Build history of the part. All positions in model axes, mm. Round coordinates to 2 decimals unless told otherwise and drop trailing zeros. Order: outer loops, then holes, each group sorted by start corner. A loop starts at its lowest first (then second) coordinate and runs counter-clockwise, first axis right, second up. Notation, with made-up numbers: M -1.75,-20.5 L 12.25,-20.5 A29 ccw 12.25,10.5 Z; hole C -31.5,4 d3. An arc over 180 degrees is marked long. One line per item, written item: value. Start each with the question number.
Item 1: Band-saw the part on B-B, the plane x = -73.5. Write the cut outline in (y, z).
Item 2: Band-saw the part on D-D, the plane x = 74.5. Write the cut outline in (y, z).
Item 3: Band-saw the part on A-A, the plane y = 117.61. Write the cut outline in (x, z), then the cut area to 3 significant figures.
Item 4: Pin check, flat tips, straight feed: pin 1 (3.5 mm diameter, centred on x = 43.36, y = -61.74, fed in from -Z); pin 2 (5.5 mm diameter, centred on x = -92.5, y = 129.72, fed in from -Z). Stop position of each tip, or through.
Item 5: Probe L1, parallel to Y at x = 86, z = 0.1; L2, parallel to Y at x = 61, z = 0.1; L3, parallel to Y at x = 23, z = 0.05. List the from-to ranges inside material, lowest first.
Item 6: Band-saw the part on C-C, the plane z = 0.1. Give the number of separate pieces and of enclosed holes in the cut face, then the cut area to 3 significant figures.
```python
from build123d import *

# Parameters (mm, degrees)
F0_R     = 2.25
F0_R_2   = 1.75
F0_R_3   = 10.5
F0_R_4   = 4.25
F0_R_5   = 2.75
F0_R_6   = 15
F1_DEPTH = 0.254


with BuildPart() as f1:
    # F0 (on Top) → F1 (new body)
    with BuildSketch(Plane.XY):
        Polygon((-17.5, -150), (92.5, -150), (102.5, -140), (102.5, -8.17), (92.5, 1.83), (58.4225, 1.83), (-7.088235, 108.588235), (-48.5, 150), (-86.5, 150), (-102.5, 134), (-102.5, -60), (-92.5, -70), (-37.5, -70), (-27.5, -80), (-27.5, -140), align=None)
        with Locations((-10.96, -138.5)):
            Circle(F0_R, mode=Mode.SUBTRACT)
        with BuildLine():
            Line((-13.21, -87.3), (-13.21, -83.3))
            ThreePointArc((-13.21, -83.3), (-10.96, -81.05), (-8.71, -83.3))
            Line((-8.71, -83.3), (-8.71, -87.3))
            ThreePointArc((-8.71, -87.3), (-10.96, -89.55), (-13.21, -87.3))
        make_face(mode=Mode.SUBTRACT)
        with Locations((-92.5, -50.28)):
            Circle(F0_R_2, mode=Mode.SUBTRACT)
        with Locations((-67.5, -38.17)):
            Circle(F0_R_3, mode=Mode.SUBTRACT)
        with Locations((-92.5, -22.78)):
            Circle(F0_R_2, mode=Mode.SUBTRACT)
        with Locations((-42.5, -50.28)):
            Circle(F0_R_2, mode=Mode.SUBTRACT)
        with Locations((-13.07, -60.17)):
            Circle(F0_R_4, mode=Mode.SUBTRACT)
        with Locations((-42.5, -22.78)):
            Circle(F0_R_2, mode=Mode.SUBTRACT)
        with Locations((21.36, -138.5)):
            Circle(F0_R, mode=Mode.SUBTRACT)
        with BuildLine():
            Line((19.11, -87.3), (19.11, -83.3))
            ThreePointArc((19.11, -83.3), (21.36, -81.05), (23.61, -83.3))
            Line((23.61, -83.3), (23.61, -87.3))
            ThreePointArc((23.61, -87.3), (21.36, -89.55), (19.11, -87.3))
        make_face(mode=Mode.SUBTRACT)
        with Locations((53.68, -138.5)):
            Circle(F0_R, mode=Mode.SUBTRACT)
        with Locations((86, -138.5)):
            Circle(F0_R, mode=Mode.SUBTRACT)
        with BuildLine():
            Line((51.43, -87.3), (51.43, -83.3))
            ThreePointArc((51.43, -83.3), (53.68, -81.05), (55.93, -83.3))
            Line((55.93, -83.3), (55.93, -87.3))
            ThreePointArc((55.93, -87.3), (53.68, -89.55), (51.43, -87.3))
        make_face(mode=Mode.SUBTRACT)
        with BuildLine():
            Line((83.75, -87.3), (83.75, -83.3))
            ThreePointArc((83.75, -83.3), (86, -81.05), (88.25, -83.3))
            Line((88.25, -83.3), (88.25, -87.3))
            ThreePointArc((88.25, -87.3), (86, -89.55), (83.75, -87.3))
        make_face(mode=Mode.SUBTRACT)
        with Locations((21.93, -60.17)):
            Circle(F0_R_4, mode=Mode.SUBTRACT)
        with Locations((43.36, -61.74)):
            Circle(F0_R_5, mode=Mode.SUBTRACT)
        with Locations((43.36, -14.6)):
            Circle(F0_R_5, mode=Mode.SUBTRACT)
        with Locations((51.43, -53.67)):
            Circle(F0_R_2, mode=Mode.SUBTRACT)
        with Locations((66.93, -38.17)):
            Circle(F0_R_6, mode=Mode.SUBTRACT)
        with Locations((90.5, -61.74)):
            Circle(F0_R_5, mode=Mode.SUBTRACT)
        with Locations((82.43, -53.67)):
            Circle(F0_R_2, mode=Mode.SUBTRACT)
        with Locations((51.43, -22.67)):
            Circle(F0_R_2, mode=Mode.SUBTRACT)
        with Locations((82.43, -22.67)):
            Circle(F0_R_2, mode=Mode.SUBTRACT)
        with Locations((90.5, -14.6)):
            Circle(F0_R_5, mode=Mode.SUBTRACT)
        with Locations((-92.5, 4.72)):
            Circle(F0_R_2, mode=Mode.SUBTRACT)
        with Locations((-91.07, 16.15)):
            Circle(F0_R_5, mode=Mode.SUBTRACT)
        with Locations((-83, 24.22)):
            Circle(F0_R_2, mode=Mode.SUBTRACT)
        with Locations((-67.5, 4.72)):
            Circle(F0_R_2, mode=Mode.SUBTRACT)
        with Locations((-52, 24.22)):
            Circle(F0_R_2, mode=Mode.SUBTRACT)
        with Locations((-92.5, 39.72)):
            Circle(F0_R_2, mode=Mode.SUBTRACT)
        with Locations((-83, 55.22)):
            Circle(F0_R_2, mode=Mode.SUBTRACT)
        with Locations((-91.07, 63.29)):
            Circle(F0_R_5, mode=Mode.SUBTRACT)
        with Locations((-92.5, 74.72)):
            Circle(F0_R_2, mode=Mode.SUBTRACT)
        with Locations((-67.5, 39.72)):
            Circle(F0_R_6, mode=Mode.SUBTRACT)
        with Locations((-52, 55.22)):
            Circle(F0_R_2, mode=Mode.SUBTRACT)
        with Locations((-67.5, 74.72)):
            Circle(F0_R_2, mode=Mode.SUBTRACT)
        with Locations((-42.5, 4.72)):
            Circle(F0_R_2, mode=Mode.SUBTRACT)
        with Locations((-43.93, 16.15)):
            Circle(F0_R_5, mode=Mode.SUBTRACT)
        with Locations((-42.5, 39.72)):
            Circle(F0_R_2, mode=Mode.SUBTRACT)
        with Locations((-43.93, 63.29)):
            Circle(F0_R_5, mode=Mode.SUBTRACT)
        with Locations((-42.5, 74.72)):
            Circle(F0_R_2, mode=Mode.SUBTRACT)
        with Locations((-92.5, 102.22)):
            Circle(F0_R_2, mode=Mode.SUBTRACT)
        with Locations((-92.5, 129.72)):
            Circle(F0_R_2, mode=Mode.SUBTRACT)
        with Locations((-67.5, 117.61)):
            Circle(F0_R_3, mode=Mode.SUBTRACT)
        with Locations((-42.5, 102.22)):
            Circle(F0_R_2, mode=Mode.SUBTRACT)
        with Locations((-42.5, 129.72)):
            Circle(F0_R_2, mode=Mode.SUBTRACT)
    extrude(amount=F1_DEPTH)


solid = f1.part
```
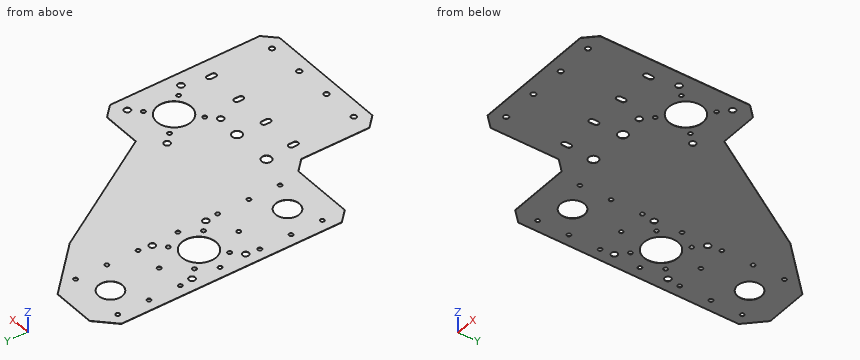
Output:
1. outline: M -70,0 L -46.79,0 L -46.79,0.25 L -70,0.25 Z; M -29.55,0 L 25.97,0 L 25.97,0.25 L -29.55,0.25 Z; M 53.47,0 L 108.99,0 L 108.99,0.25 L 53.47,0.25 Z; M 126.23,0 L 150,0 L 150,0.25 L 126.23,0.25 Z
2. outline: M -150,0 L -51.12,0 L -51.12,0.25 L -150,0.25 Z; M -25.22,0 L 1.83,0 L 1.83,0.25 L -25.22,0.25 Z
3. outline: M -102.5,0 L -78,0 L -78,0.25 L -102.5,0.25 Z; M -57,0 L -16.11,0 L -16.11,0.25 L -57,0.25 Z
3. area: 16.6 mm²
4. pin 1: passes through
4. pin 2: stops at z = 0
5. L1: y = -150 to -140.75, -136.25 to -89.55, -81.05 to 1.83
5. L2: y = -150 to -51.95, -24.39 to 1.83
5. L3: y = -150 to -140.04, -136.96 to -88.84, -81.76 to -64.28, -56.06 to 59.56
6. separate pieces: 1
6. enclosed holes: 46
6. area: 38,800 mm²
